Can you work these out from the model? Positions are in its coordinate system, mm. Round coordinates to 2 decimals unless told otherwise and drop trailing zeros. Write each loop counter-clockwise with the first axis right and the second up, starting at its lowest first coordinate (ties: lowest second). Pieces come first, ordered by that corner, then holes. Notation, with made-up numbers: M 27,-5.75 L 36,-5.75 A25 ccw 36,6.25 Z; hole C -36,44.5 d2. An arc over 180 degrees is marked long. Answer in a Markdown table with one row per item. Add a question column.
(1) Suppose I cut it at D-D, the plane z = 0.8. Write out the boundary of the cut face in (x, y).
(2) Suppose I cut it at A-A, the plane x = -3.75. Write out the boundary of the cut face in (y, z).
(3) If I drill on probe 1 along X at (y, z) = (7.5, 0); probe 2 along Z at (x, y) = (3.75, 8); probe 3 along Z at (x, y) = (1.25, 1.5), over which ranges is the centre line in solid material (lowest first)?
(4) Suppose I cut it at B-B, the plane y = 3.5. Write out the boundary of the cut face in (x, z).
(5) Suppose I cut it at C-C, the plane z = 0. Count the separate pieces of the cut face and the enclosed holes in it, then the cut area to 3 significant figures.
from build123d import *

# Parameters (mm, degrees)
SKETCH_1_W      = 10
SKETCH_1_H      = 2
SKETCH_1_W_2    = 0.5
SKETCH_1_H_2    = 0.5
EXTRUDE_1_DEPTH = 7
SKETCH_2_W      = 10
SKETCH_2_H      = 2
SKETCH_2_R      = 0.353553391
EXTRUDE_2_DEPTH = 2
CHAMFER_1_SIZE  = 0.5


with BuildPart() as part:
    # Эскиз1 → Бобышка-Вытянуть1 (new body)
    with BuildSketch(Plane(origin=(0, 0, 0), x_dir=(1, 0, 0), z_dir=(0, 1, 0))):
        Rectangle(SKETCH_1_W, SKETCH_1_H)
        with Locations((-3.75, 0)):
            Rectangle(SKETCH_1_W_2, SKETCH_1_H_2, mode=Mode.SUBTRACT)
        with Locations((3.75, 0)):
            Rectangle(SKETCH_1_W_2, SKETCH_1_H_2, mode=Mode.SUBTRACT)
        with Locations((-1.25, 0)):
            Rectangle(SKETCH_1_W_2, SKETCH_1_H_2, mode=Mode.SUBTRACT)
        with Locations((1.25, 0)):
            Rectangle(SKETCH_1_W_2, SKETCH_1_H_2, mode=Mode.SUBTRACT)
    extrude(amount=EXTRUDE_1_DEPTH)

    # Эскиз2 → Бобышка-Вытянуть2 (add)
    with BuildSketch(Plane(origin=(0, 7, 0), x_dir=(1, 0, 0), z_dir=(0, 1, 0))):
        Rectangle(SKETCH_2_W, SKETCH_2_H)
        with Locations((-3.75, 0)):
            Circle(SKETCH_2_R, mode=Mode.SUBTRACT)
        with Locations((-1.25, 0)):
            Circle(SKETCH_2_R, mode=Mode.SUBTRACT)
        with Locations((1.25, 0)):
            Circle(SKETCH_2_R, mode=Mode.SUBTRACT)
        with Locations((3.75, 0)):
            Circle(SKETCH_2_R, mode=Mode.SUBTRACT)
    extrude(amount=EXTRUDE_2_DEPTH)

    # Фаска1
    chamfer_1_edges = [part.edges().sort_by_distance(p)[0] for p in [
        (5, 4.5, 1),
        (-5, 4.5, 1),
        (-5, 4.5, -1),
        (5, 4.5, -1),
    ]]
    chamfer(chamfer_1_edges, length=CHAMFER_1_SIZE)


solid = part.part
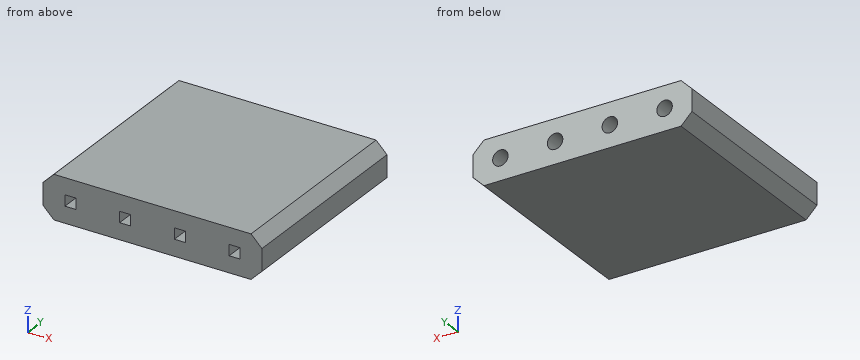
Calculated:
| question | item | result |
|---|---|---|
| 1 | outline | M -4.7,0 L 4.7,0 L 4.7,9 L -4.7,9 Z |
| 2 | outline | M 0,-1 L 9,-1 L 9,-0.35 L 7,-0.35 L 7,-0.25 L 0,-0.25 Z; M 0,0.25 L 7,0.25 L 7,0.35 L 9,0.35 L 9,1 L 0,1 Z |
| 3 | probe 1 | -5 to -4.1, -3.4 to -1.6, -0.9 to 0.9, 1.6 to 3.4, 4.1 to 5 |
| 3 | probe 2 | -1 to -0.35, 0.35 to 1 |
| 3 | probe 3 | -1 to -0.25, 0.25 to 1 |
| 4 | outline | M -5,-0.5 L -4.5,-1 L 4.5,-1 L 5,-0.5 L 5,0.5 L 4.5,1 L -4.5,1 L -5,0.5 Z; hole M -4,-0.25 L -3.5,-0.25 L -3.5,0.25 L -4,0.25 Z; hole M -1.5,-0.25 L -1,-0.25 L -1,0.25 L -1.5,0.25 Z; hole M 1,-0.25 L 1.5,-0.25 L 1.5,0.25 L 1,0.25 Z; hole M 3.5,-0.25 L 4,-0.25 L 4,0.25 L 3.5,0.25 Z |
| 5 | separate pieces | 5 |
| 5 | enclosed holes | 0 |
| 5 | area | 70.3 mm² |
